The model under review builds one solid part; all positions refer to its coordinate system, in mm. Face numbers are marked on the shaded views. Round coordinates to 2 decimals unless told otherwise and drop trailing zeros. Write each loop counter-clockwise with the first axis right and the second up, starting at its lowest first coordinate (ties: lowest second). Pieces come first, ordered by that corner, then holes. Notation, with made-up numbers: (50, 2) -> (67, 2) arc R18 ccw to (67, 15) -> close; hole circle Ø9 at (-6, 50.25). An arc over 180 degrees is marked (long way). Return JSON: item names as keys, results as strings. Group by question number.
1. Clearance check with flat-ended pins moving along their axes: P1, Ø4, axis at y = 3, z = 4, coming from the +X side; P2, Ø1.5, axis at x = 1, y = 7, coming from the -Z side; P3, Ø1.5, axis at y = 3.5, z = 1, coming from the -X side. State where each tip first meets the part, or that it passes through.
2. Take a section at B-B, the plane z = 5. Write out the cut boundary in (x, y), then the cut area to 3 significant figures.
3. For line 1 along Y through (x, z) = (0, 5.5); line 2 along Y through (x, z) = (-2.25, 7); line 3 along X through (y, z) = (-4, 4), list the stretches that pass through material, from the lowest coordinate up. Write a range as from..to.
4. Take a section at A-A, the plane x = 0. Write out the cut boundary in (y, z), then the cut area to 3 significant figures.
5. Mouldability with a two-part tool opening along Y and no side actions: class the marked faces 1, 2, 3 and 4 as pulls with the +Y half, pulls with the -Y half, needs draft (parallel to the pull), parting line crosses it, or undercut.
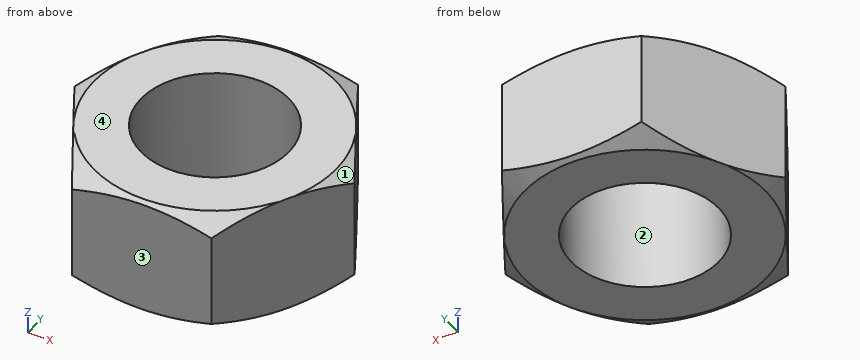
from build123d import *

# Parameters (mm, degrees)
BOSS_EXTRUDE1_DEPTH = 8
SKETCH2_OUTSIDE_W   = 60.666
SKETCH2_OUTSIDE_H   = 58.946
SKETCH2_OUTSIDE_R   = 8.199202844
CUT_EXTRUDE1_DEPTH  = 10
CUT_EXTRUDE1_TAPER  = 60
SKETCH3_OUTSIDE_W   = 29.488
SKETCH3_OUTSIDE_H   = 27.768
SKETCH3_OUTSIDE_R   = 8.172152793
CUT_EXTRUDE2_DEPTH  = 1
CUT_EXTRUDE2_TAPER  = 60
SKETCH4_R           = 5
CUT_EXTRUDE3_DEPTH  = 8


with BuildPart() as part:
    # Sketch1 → Boss-Extrude1 (new body)
    with BuildSketch(Plane.XY):
        Polygon((9.359699903, 0), (4.68, 8.5), (-4.68, 8.5), (-9.36, -0.105997779), (-4.68, -8.5), (4.68, -8.5), align=None)
    extrude(amount=BOSS_EXTRUDE1_DEPTH)

    # Sketch2 outside → Cut-Extrude1 (cut)
    with BuildSketch(Plane.XY.offset(8)):
        Rectangle(SKETCH2_OUTSIDE_W, SKETCH2_OUTSIDE_H)
        Circle(SKETCH2_OUTSIDE_R, mode=Mode.SUBTRACT)
    extrude(amount=-CUT_EXTRUDE1_DEPTH, taper=CUT_EXTRUDE1_TAPER, mode=Mode.SUBTRACT)

    # Sketch3 outside → Cut-Extrude2 (cut)
    with BuildSketch(Plane(origin=(0, 0, 0), x_dir=(-1, 0, 0), z_dir=(0, 0, -1))):
        Rectangle(SKETCH3_OUTSIDE_W, SKETCH3_OUTSIDE_H)
        Circle(SKETCH3_OUTSIDE_R, mode=Mode.SUBTRACT)
    extrude(amount=-CUT_EXTRUDE2_DEPTH, taper=CUT_EXTRUDE2_TAPER, mode=Mode.SUBTRACT)

    # Sketch4 → Cut-Extrude3 (cut)
    with BuildSketch(Plane.XY.offset(8)):
        Circle(SKETCH4_R)
    extrude(amount=-CUT_EXTRUDE3_DEPTH, mode=Mode.SUBTRACT)


solid = part.part
Output:
{
 "1": {"P1": "stops at x = 8.81", "P2": "stops at z = 0", "P3": "stops at x = -7.81"},
 "2": {"outline": "(-9.36, -0.11) -> (-4.68, -8.5) -> (4.68, -8.5) -> (9.36, 0) -> (4.68, 8.5) -> (-4.68, 8.5) -> close; hole circle Ø10 at (0, 0)", "area": "160 mm^2"},
 "3": {"line 1": "y = -8.5..-5, 5..8.5", "line 2": "y = -8.5..-4.47, 4.47..8.5", "line 3": "x = -7.19..-3, 3..7.16"},
 "4": {"outline": "(-8.5, 0.19) -> (-8.17, 0) -> (-5, 0) -> (-5, 8) -> (-8.2, 8) -> (-8.5, 7.83) -> close; (5, 0) -> (8.17, 0) -> (8.5, 0.19) -> (8.5, 7.83) -> (8.2, 8) -> (5, 8) -> close", "area": "55.9 mm^2"},
 "5": {"face 1": "parting line crosses it", "face 2": "undercut", "face 3": "pulls with the -Y half", "face 4": "needs draft"}
}
